Geometry: see drawing. Coordinates: mm, zero at the bounding-box minimum. Round coordinates to 2 decimals unless told otherwise and drop trailing zeros. Order: outer loops, then holes, each group sorted by start corner. A loop starts at its lowest first (then second) coordinate and runs counter-clockwise, first axis right, second up. Notation, with made-up numbers: (72, 41) -> (124, 41) arc R15 ccw to (124, 56) -> close; hole circle Ø3 at (-5, 59). An arc over 180 degrees is marked (long way). Put each result on its own line as item: value.
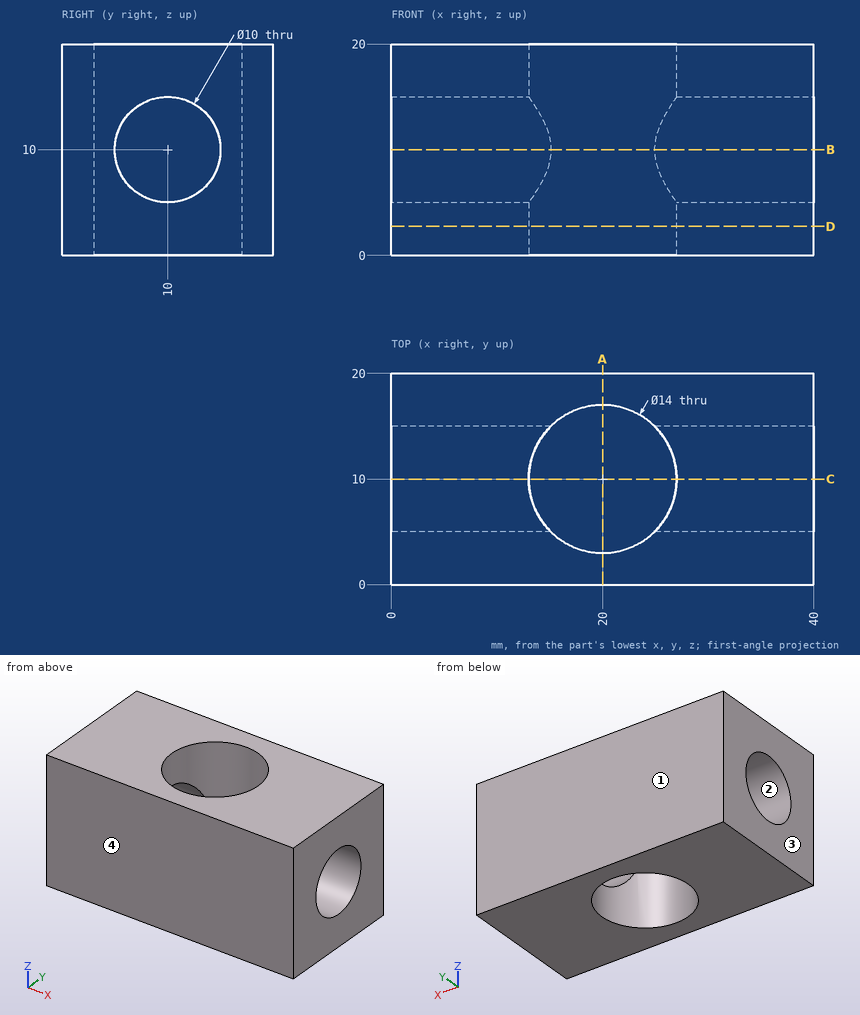
1. Material intervals for probe 1 along Y at (x, z) = (33.75, 10); probe 2 along Y at (x, z) = (20, 12); probe 3 along X at (y, z) = (10, 16.25), sorted ascending.
Ans:
probe 1: 0 to 5, 15 to 20
probe 2: 0 to 3, 17 to 20
probe 3: 0 to 13, 27 to 40
2. Cut plane A-A on x = 20. Return loops of the section in (y, z).
Ans:
outline: (0, 0) -> (3, 0) -> (3, 20) -> (0, 20) -> close; (17, 0) -> (20, 0) -> (20, 20) -> (17, 20) -> close
3. Cut plane C-C on y = 10. Return loops of the section in (x, z), and give its area (3 significant figures).
Ans:
outline: (0, 0) -> (13, 0) -> (13, 5) -> (0, 5) -> close; (0, 15) -> (13, 15) -> (13, 20) -> (0, 20) -> close; (27, 0) -> (40, 0) -> (40, 5) -> (27, 5) -> close; (27, 15) -> (40, 15) -> (40, 20) -> (27, 20) -> close
area: 260 mm²
4. Cut plane D-D on z = 2.75. Return loops of the section in (x, y), and give its area (3 significant figures).
Ans:
outline: (0, 0) -> (40, 0) -> (40, 20) -> (0, 20) -> close; hole circle Ø14 at (20, 10)
area: 646 mm²
5. Draft query along Y for the marked faces 1, 2, 3 and 4. Return one class per face: +Y half, -Y half, draft (parallel to the pull), parting line (faces both ways), or undercut.
Ans:
face 1: +Y half
face 2: undercut
face 3: draft
face 4: -Y half
6. Cut plane B-B on z = 10. Return loops of the section in (x, y), and give its area (3 significant figures).
Ans:
outline: (0, 0) -> (40, 0) -> (40, 5) -> (24.9, 5) arc R7 cw to (15.1, 5) -> (0, 5) -> close; (0, 15) -> (15.1, 15) arc R7 cw to (24.9, 15) -> (40, 15) -> (40, 20) -> (0, 20) -> close
area: 373 mm²
